Verification items for the finished model (mm, model axes). Face numbers are marked on the shaded views. A direction names the side the tool comes from. Coordinates: 2 decimals unless noted, no trailing zeros. Order: outer loops, then holes, each group sorted by start corner. A loop starts at its lowest first (then second) coordinate and runs counter-clockwise, first axis right, second up. Notation, with made-up numbers: (80, 3) -> (88, 3) arc R29 ccw to (88, 23) -> close; hole circle Ø8 at (-10, -25). An arc over 180 degrees is marked (long way). Use CSV: the item, a comma, the result in double quotes. Start each with the question number.
1) Release check for a two-part mould opening along Y. For the marked faces 1, 2, 3 and 4 record: released by +Y, released by -Y, zero draft, split by the parting line, or undercut.
2) Sectioned sample at C-C on y = 22. Record the boundary of the cut face in (x, z).
3) Sectioned sample at B-B on z = 3.7. Give the number of separate pieces and of enclosed holes in the cut face, then the cut area to 3 significant figures.
4) Sectioned sample at A-A on y = 7. Record the boundary of the cut face in (x, z), then the cut area to 3 significant figures.
5) Scan lines: line 1 along Y through (x, z) = (-15, 3.9); line 2 along X through (y, z) = (-44, 5.2); line 3 along Y through (x, z) = (-44, 3.7). Record each from-to range of solid material in increasing order.
6) Go/stop test with flat-tipped pins: pin 1 (2 mm diameter, centred on x = 15, y = -15, fed in from +Z); pin 2 (1.7 mm diameter, centred on y = 11, z = 3, fed in from +X); pin 3 (1.7 mm diameter, centred on y = 37.5, z = 4, fed in from +X); pin 4 (3 mm diameter, centred on x = 35, z = 2.5, fed in from -Y). Record where each tip stops, or that it passes through.
7) Tool access check on the marked faces 5, 6, 7 and 8. Record the directions out of +Z, -Z, +X, -X, +Y, -Y that give a thin tool (end or side, any length) a straight path to the whole face; none if there is none.
from build123d import *

# Parameters (mm, degrees)
SKETCH1_R           = 1.25
SKETCH1_RX          = 7.495001668
SKETCH1_RY          = 2.505000234
SKETCH1_RX_2        = 10.410152117
SKETCH1_RY_2        = 2.505
BOSS_EXTRUDE1_DEPTH = 5.8


with BuildPart() as part:
    # Sketch1 → Boss-Extrude1 (new body)
    with BuildSketch(Plane.XY):
        with BuildLine():
            Line((-16, 20), (-8.99, 20))
            ThreePointArc((-8.99, 20), (-5.815090552, 21.315090552), (-4.5, 24.49))
            Line((-4.5, 24.49), (-4.5, 44))
            ThreePointArc((-4.5, 44), (-3.181980515, 47.181980515), (0, 48.5))
            ThreePointArc((0, 48.5), (3.181980515, 47.181980515), (4.5, 44))
            Line((4.5, 44), (4.5, 24.49))
            ThreePointArc((4.5, 24.49), (5.815090552, 21.315090552), (8.99, 20))
            Line((8.99, 20), (16, 20))
            ThreePointArc((16, 20), (18.828427125, 18.828427125), (20, 16))
            Line((20, 16), (20, 8.99))
            ThreePointArc((20, 8.99), (21.315090552, 5.815090552), (24.49, 4.5))
            Line((24.49, 4.5), (50, 4.5))
            ThreePointArc((50, 4.5), (54.5, 0), (50, -4.5))
            Line((50, -4.5), (24.49, -4.5))
            ThreePointArc((24.49, -4.5), (21.315090552, -5.815090552), (20, -8.99))
            Line((20, -8.99), (20, -16))
            ThreePointArc((20, -16), (18.828427125, -18.828427125), (16, -20))
            Line((16, -20), (8.99, -20))
            ThreePointArc((8.99, -20), (5.815090552, -21.315090552), (4.5, -24.49))
            Line((4.5, -24.49), (4.5, -44))
            ThreePointArc((4.5, -44), (3.181980515, -47.181980515), (0, -48.5))
            ThreePointArc((0, -48.5), (-3.181980515, -47.181980515), (-4.5, -44))
            Line((-4.5, -44), (-4.5, -24.49))
            ThreePointArc((-4.5, -24.49), (-5.815090552, -21.315090552), (-8.99, -20))
            Line((-8.99, -20), (-16, -20))
            ThreePointArc((-16, -20), (-18.828427125, -18.828427125), (-20, -16))
            Line((-20, -16), (-20, -8.99))
            ThreePointArc((-20, -8.99), (-21.315090552, -5.815090552), (-24.49, -4.5))
            Line((-24.49, -4.5), (-50, -4.5))
            ThreePointArc((-50, -4.5), (-54.5, 0), (-50, 4.5))
            Line((-50, 4.5), (-24.49, 4.5))
            ThreePointArc((-24.49, 4.5), (-21.315090552, 5.815090552), (-20, 8.99))
            Line((-20, 8.99), (-20, 16))
            ThreePointArc((-20, 16), (-18.828427125, 18.828427125), (-16, 20))
        make_face()
        with Locations((0, 44)):
            Circle(SKETCH1_R, mode=Mode.SUBTRACT)
        with Locations((-15, 15)):
            Circle(SKETCH1_R, mode=Mode.SUBTRACT)
        with Locations(Location((15, 15, 0), (0, 0, 180))):
            Circle(SKETCH1_R, mode=Mode.SUBTRACT)
        with Locations((15, -15)):
            Circle(SKETCH1_R, mode=Mode.SUBTRACT)
        with Locations(Location((-15, -15, 0), (0, 0, 180))):
            Circle(SKETCH1_R, mode=Mode.SUBTRACT)
        with Locations((-50, 0)):
            Circle(SKETCH1_R, mode=Mode.SUBTRACT)
        with Locations(Location((50, 0, 0), (0, 0, 180))):
            Circle(SKETCH1_R, mode=Mode.SUBTRACT)
        with Locations(Location((0, -44, 0), (0, 0, 180))):
            Circle(SKETCH1_R, mode=Mode.SUBTRACT)
        with Locations(Location((-0.004999676, 32.005), (0, 0, 89.961779812))):
            Ellipse(SKETCH1_RX, SKETCH1_RY, mode=Mode.SUBTRACT)
        with Locations(Location((-0.004999676, -32.005), (0, 0, -89.961779812))):
            Ellipse(SKETCH1_RX, SKETCH1_RY, mode=Mode.SUBTRACT)
        with Locations(Location((-34.90982111, 0.001514413), (0, 0, 0.005750064))):
            Ellipse(SKETCH1_RX_2, SKETCH1_RY_2, mode=Mode.SUBTRACT)
        with Locations(Location((34.90982111, 0.001514413), (0, 0, 179.994249936))):
            Ellipse(SKETCH1_RX_2, SKETCH1_RY_2, mode=Mode.SUBTRACT)
        with BuildLine():
            Line((9.99479618, -11.99479618), (-9.99479618, -11.99479618))
            ThreePointArc((-9.99479618, -11.99479618), (-11.409009742, -11.409009742), (-11.99479618, -9.99479618))
            Line((-11.99479618, -9.99479618), (-11.99479618, 9.99479618))
            ThreePointArc((-11.99479618, 9.99479618), (-11.409009742, 11.409009742), (-9.99479618, 11.99479618))
            Line((-9.99479618, 11.99479618), (9.99479618, 11.99479618))
            ThreePointArc((9.99479618, 11.99479618), (11.409009742, 11.409009742), (11.99479618, 9.99479618))
            Line((11.99479618, 9.99479618), (11.99479618, -9.99479618))
            ThreePointArc((11.99479618, -9.99479618), (11.409009742, -11.409009742), (9.99479618, -11.99479618))
        make_face(mode=Mode.SUBTRACT)
    extrude(amount=BOSS_EXTRUDE1_DEPTH)


solid = part.part
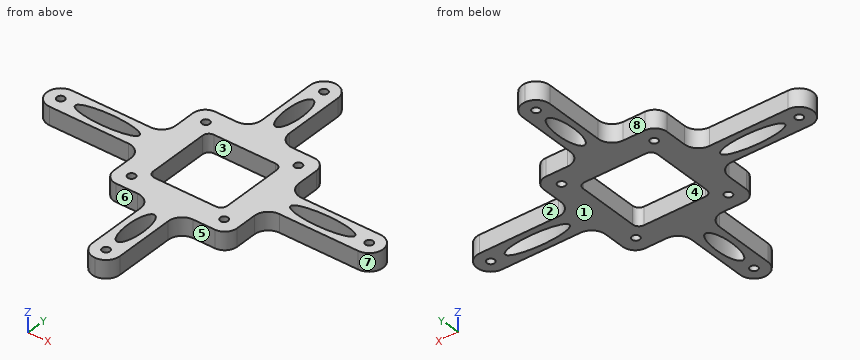
Answers follow:
1,face 1,"zero draft"
1,face 2,"released by +Y"
1,face 3,"undercut"
1,face 4,"undercut"
2,outline,"(-5.25, 0) -> (5.25, 0) -> (5.25, 5.8) -> (-5.25, 5.8) -> close"
3,separate pieces,"1"
3,enclosed holes,"13"
3,area,"1,830 mm²"
4,outline,"(-20.47, 0) -> (-11.99, 0) -> (-11.99, 5.8) -> (-20.47, 5.8) -> close; (11.99, 0) -> (20.47, 0) -> (20.47, 5.8) -> (11.99, 5.8) -> close"
4,area,"98.3 mm²"
5,line 1,"y = -20 to -16.25, -13.75 to 13.75, 16.25 to 20"
5,line 2,"x = -4.5 to -1.25, 1.25 to 4.5"
5,line 3,"y = -4.5 to -1.22, 1.22 to 4.5"
6,pin 1,"passes through"
6,pin 2,"stops at x = 20"
6,pin 3,"stops at x = 4.5"
6,pin 4,"stops at y = -4.5"
7,face 5,"+Z, -Z, +X, -Y"
7,face 6,"+Z, -Z, -X, -Y"
7,face 7,"+Z, -Z, +X"
7,face 8,"+Z, -Z, -X, +Y"
